For this review, take the finished solid that the model builds, in its own axes (mm). A direction names the side the tool comes from. Round coordinates to 2 decimals unless told otherwise and drop trailing zeros. Write each loop counter-clockwise with the first axis right and the second up, starting at its lowest first coordinate (ties: lowest second). Pieces come first, ordered by that corner, then holes.
from build123d import *

# Parameters (mm, degrees)
BOSS_EXTRUDE1_DEPTH = 430
SKETCH4_R           = 8.5
CUT_EXTRUDE2_DEPTH  = 1.5
LPATTERN1_COUNT     = 4
LPATTERN1_PITCH     = 35


with BuildPart() as part:
    # Sketch1 → Boss-Extrude1 (new body)
    with BuildSketch(Plane(origin=(0, 0, 0), x_dir=(1, 0, 0), z_dir=(0, 1, 0))):
        with BuildLine():
            Line((-35.152535823, 171.433075062), (35.152535823, 171.433075062))
            ThreePointArc((35.152535823, 171.433075062), (0, -175), (-35.152535823, 171.433075062))
        make_face()
        with BuildLine():
            ThreePointArc((-35, 169.933075062), (0, -173.5), (35, 169.933075062))
            Line((35, 169.933075062), (-35, 169.933075062))
        make_face(mode=Mode.SUBTRACT)
    extrude(amount=BOSS_EXTRUDE1_DEPTH)

    # Sketch4 → Cut-Extrude2 (cut)
    with BuildSketch(Plane(origin=(0, 0, -171.433075062), x_dir=(-1, 0, 0), z_dir=(0, 0, -1))):
        with Locations((-17.5, 401)):
            Circle(SKETCH4_R)
        with Locations((17.5, 401)):
            Circle(SKETCH4_R)
    cut_extrude2 = extrude(amount=-CUT_EXTRUDE2_DEPTH, mode=Mode.SUBTRACT)

    # LPattern1: Cut-Extrude2 ×4
    with Locations(*[(0, -i * LPATTERN1_PITCH, 0) for i in range(1, LPATTERN1_COUNT)]):
        add(cut_extrude2, mode=Mode.SUBTRACT)


solid = part.part
(1) For faces 4 (the face through (-7.136, 211.99, 173.353)), 5 (the face through (18.607, 374.428, -170.694)), list the 3-axis set-ups (+Z, -Z, +X, -X, +Y, -Y) from which the entire face can be reached by the end or side of a thin tool; tool diameter is ignored.
Geometry check:
face 4: +Y, -Y
face 5: -Z
(2) We need section B-B, the plane x = -17.5. Give the boundary of the cut face in (y, z), and give its area (3 significant figures).
Geometry check:
outline: (0, -171.43) - (287.5, -171.43) - (287.5, -169.93) - (0, -169.93) - close; (0, 172.62) - (430, 172.62) - (430, 174.12) - (0, 174.12) - close; (304.5, -171.43) - (322.5, -171.43) - (322.5, -169.93) - (304.5, -169.93) - close; (339.5, -171.43) - (357.5, -171.43) - (357.5, -169.93) - (339.5, -169.93) - close; (374.5, -171.43) - (392.5, -171.43) - (392.5, -169.93) - (374.5, -169.93) - close; (409.5, -171.43) - (430, -171.43) - (430, -169.93) - (409.5, -169.93) - close
area: 1,190 mm2
(3) We need section A-A, the plane y = 296. Give the boundary of the cut face in (x, z).
Geometry check:
outline: (-35.15, -171.43) - (-26, -171.43) - (-26, -169.93) - (-35, -169.93) arc R173.5 cw (long way) to (35, -169.93) - (26, -169.93) - (26, -171.43) - (35.15, -171.43) arc R175 ccw (long way) to start; (-9, -171.43) - (9, -171.43) - (9, -169.93) - (-9, -169.93) - close
(4) For line 1 along Y through (x, z) = (-17.5, -170.95); line 2 along Z through (x, y) = (77, 383.5); line 3 along X through (y, z) = (283, -44.5), list the stretches that pass through material, from the lowest coordinate up.
Geometry check:
line 1: y = 0 to 287.5, 304.5 to 322.5, 339.5 to 357.5, 374.5 to 392.5, 409.5 to 430
line 2: z = -157.15 to -155.48, 155.48 to 157.15
line 3: x = -169.25 to -167.7, 167.7 to 169.25
(5) Mouldability with a two-part tool opening along Y and no side actions: class faces 1 (the face through (0, 212, -169.933)), 2 (the face through (18.607, 304.428, -170.694)), 3 (the face through (156.4, 430, -76)) as pulls with the +Y half, pulls with the -Y half, needs draft (parallel to the pull), parting line crosses it, or undercut.
Geometry check:
face 1: needs draft
face 2: undercut
face 3: pulls with the +Y half
(6) For pin 1 Ø1.5 at (y, z) = (282, 27) entering from -X; pin 2 Ø15.5 at (x, y) = (-17.5, 331) entering from +Z; pin 3 Ø15.5 at (x, y) = (-17.5, 366) entering from -Z, all flat-tipped, find the tip position at first contact; note any pin that passes through.
Geometry check:
pin 1: stops at x = -173.02
pin 2: stops at z = 174.73
pin 3: stops at z = 171.65
(7) We need section C-C, the plane z = 30. Give the boundary of the cut face in (x, y), and give its area (3 significant figures).
Geometry check:
outline: (-172.41, 0) - (-170.89, 0) - (-170.89, 430) - (-172.41, 430) - close; (170.89, 0) - (172.41, 0) - (172.41, 430) - (170.89, 430) - close
area: 1,310 mm2
(8) We need section D-D, the plane x = 122. Give the boundary of the cut face in (y, z).
Geometry check:
outline: (0, -125.46) - (430, -125.46) - (430, -123.36) - (0, -123.36) - close; (0, 123.36) - (430, 123.36) - (430, 125.46) - (0, 125.46) - close
